Input: part model. Units: mm. Frame: model coordinates. A direction names the side the tool comes from. Round coordinates to 2 decimals unless told otherwise and drop trailing zeros. Loops run counter-clockwise (first coordinate to the right, second up) from the corner with the lowest first, then second, coordinate; pieces in that order, holes last. Notation, with made-up numbers: M 29.25,31 L 80.25,31 A10 cw 80.25,42 Z; hole C 54,56 d9. An arc over 180 degrees is marked long. Return JSON: item names as keys, results as strings. Group by question number.
1) Section B-B (x = 16.5). Output: boundary loops of the cut face in (y, z).
2) Mould query, pull axis X, two halves, no side actions, for faces 4 (the face through (25.792, 1264.618, 375.666)), 5 (the face through (282.514, -527.59, 112.7)), 6 (the face through (-250.886, -524.39, 112.7)), 7 (the face through (-70.49, 714.704, 375.666)). Classes: +X half, -X half, draft (parallel to the pull), parting line (faces both ways), or undercut.
3) Section A-A (z = 90.5). Output: boundary loops of the cut face in (x, y), plus the area to 3 significant figures.
4) Contact query for flat-ended pins moving along their axis: P1, Ø3, axis at y = 361.5, z = 664, coming from the +X side; P2, Ø4, axis at x = -148, y = -435.5, coming from the +Z side; P3, Ø1.5, axis at x = -245, z = 192.5, coming from the +Y side (3 decimals). Output: stop coordinate, or through.
5) Material intervals for line 1 (Z direction, x = -296.5, y = 27.5); line 2 (X direction, y = 812, z = 674); line 3 (Y direction, x = -72.5, z = 339.5), sorted ascending. Write a range as from..to.
6) Access query for faces 1 (the face through (-363.586, 389, 206)), 2 (the face through (-220, -61, 228.6)), 3 (the face through (250, 502.71, 492)). Directions: +Z, -Z, +X, -X, +Y, -Y. A direction counts if a zero-diameter tool reaches every point of the face in a straight line with its end or side. Return the directions, or none.
7) Section C-C (y = 793). Output: boundary loops of the cut face in (x, z), plus the area to 3 significant figures.
8) Section D-D (z = 345.5). Output: boundary loops of the cut face in (x, y), plus the area to 3 significant figures.
from build123d import *

# Parameters (mm, degrees)
F0_W     = 177.8
F0_H     = 1143
F1_DEPTH = 228.6
F2_DEPTH = 762
F4_DEPTH = 177.8


with BuildPart() as f1:
    # F0 (on Top) → F1 (new body)
    with BuildSketch(Plane.XY):
        Polygon((398.4137039741, -411.6901900116), (398.4137039741, 502.7098099884), (106.3137039741, 502.7098099884), (106.3137039741, -640.2901900116), (169.8137039741, -640.2901900116), align=None)
        with BuildLine():
            Line((398.4137039741, 883.7098099884), (207.9137039741, 883.7098099884))
            ThreePointArc((207.9137039741, 883.7098099884), (17.4137039741, 693.2098099884), (-173.0862960259, 883.7098099884))
            Line((-173.0862960259, 883.7098099884), (-363.5862960259, 883.7098099884))
            Line((-363.5862960259, 883.7098099884), (-363.5862960259, 502.7098099884))
            Line((-363.5862960259, 502.7098099884), (-71.4862960259, 502.7098099884))
            Line((-71.4862960259, 502.7098099884), (106.3137039741, 502.7098099884))
            Line((106.3137039741, 502.7098099884), (398.4137039741, 502.7098099884))
            Line((398.4137039741, 502.7098099884), (398.4137039741, 883.7098099884))
        make_face()
        Polygon((-71.4862960259, 502.7098099884), (-363.5862960259, 502.7098099884), (-363.5862960259, -411.6901900116), (-134.9862960259, -640.2901900116), (-71.4862960259, -640.2901900116), align=None)
        with Locations((17.4137039741, -68.7901900116)):
            Rectangle(F0_W, F0_H)
        with BuildLine():
            ThreePointArc((-173.0862960259, 883.7098099884), (17.4137039741, 1074.2098099884), (207.9137039741, 883.7098099884))
            Line((207.9137039741, 883.7098099884), (398.4137039741, 883.7098099884))
            ThreePointArc((398.4137039741, 883.7098099884), (17.4137039741, 1264.7098099884), (-363.5862960259, 883.7098099884))
            Line((-363.5862960259, 883.7098099884), (-173.0862960259, 883.7098099884))
        make_face()
    extrude(amount=F1_DEPTH)

    # F0 (on Top) → F2 (join)
    with BuildSketch(Plane.XY):
        with BuildLine():
            Line((398.4137039741, 883.7098099884), (207.9137039741, 883.7098099884))
            ThreePointArc((207.9137039741, 883.7098099884), (17.4137039741, 693.2098099884), (-173.0862960259, 883.7098099884))
            Line((-173.0862960259, 883.7098099884), (-363.5862960259, 883.7098099884))
            Line((-363.5862960259, 883.7098099884), (-363.5862960259, 502.7098099884))
            Line((-363.5862960259, 502.7098099884), (-71.4862960259, 502.7098099884))
            Line((-71.4862960259, 502.7098099884), (106.3137039741, 502.7098099884))
            Line((106.3137039741, 502.7098099884), (398.4137039741, 502.7098099884))
            Line((398.4137039741, 502.7098099884), (398.4137039741, 883.7098099884))
        make_face()
        with Locations((17.4137039741, -68.7901900116)):
            Rectangle(F0_W, F0_H)
        with BuildLine():
            ThreePointArc((-173.0862960259, 883.7098099884), (17.4137039741, 1074.2098099884), (207.9137039741, 883.7098099884))
            Line((207.9137039741, 883.7098099884), (398.4137039741, 883.7098099884))
            ThreePointArc((398.4137039741, 883.7098099884), (17.4137039741, 1264.7098099884), (-363.5862960259, 883.7098099884))
            Line((-363.5862960259, 883.7098099884), (-173.0862960259, 883.7098099884))
        make_face()
    extrude(amount=F2_DEPTH)

    # F3 (on face) → F4 (cut)
    with BuildSketch(Plane.YZ.offset(106.3137039741)):
        Polygon((-640.2901900116, 762), (-640.2901900116, 228.6), (502.7098099884, 762), align=None)
    extrude(amount=-F4_DEPTH, mode=Mode.SUBTRACT)


solid = f1.part
Returned:
{
 "1": {"outline": "M -640.29,0 L 693.21,0 L 693.21,762 L 502.71,762 L -640.29,228.6 Z; M 1074.21,0 L 1264.71,0 L 1264.71,762 L 1074.21,762 Z"},
 "2": {"face 4": "parting line", "face 5": "+X half", "face 6": "-X half", "face 7": "undercut"},
 "3": {"outline": "M -363.59,-411.69 L -134.99,-640.29 L 169.81,-640.29 L 398.41,-411.69 L 398.41,883.71 A381 ccw -363.59,883.71 Z; hole C 17.41,883.71 d381", "area": "1,220,000 mm^2"},
 "4": {"P1": "stops at x = 106.31", "P2": "stops at z = 228.6", "P3": "stops at y = 1160.645"},
 "5": {"line 1": "z = 0..228.6", "line 2": "x = -363.59..-159.07, 193.9..398.41", "line 3": "y = 502.71..715.76, 1051.66..1253.95"},
 "6": {"face 1": "+Z, -Z, -X, +Y, -Y", "face 2": "+Z, -X, -Y", "face 3": "+Z, +X, -Y"},
 "7": {"outline": "M -363.59,0 L -150.1,0 L -150.1,762 L -363.59,762 Z; M 184.93,0 L 398.41,0 L 398.41,762 L 184.93,762 Z", "area": "325,000 mm^2"},
 "8": {"outline": "M -363.59,502.71 L -71.49,502.71 L -71.49,-389.79 L 106.31,-389.79 L 106.31,502.71 L 398.41,502.71 L 398.41,883.71 A381 ccw -363.59,883.71 Z; hole C 17.41,883.71 d381", "area": "563,000 mm^2"}
}
